Part model, mm, in its own coordinate system. A direction names the side the tool comes from. Round coordinates to 2 decimals unless told otherwise and drop trailing zeros. Loops run counter-clockwise (first coordinate to the right, second up) from the corner with the lowest first, then second, coordinate; pieces in that order, holes last. Notation, with made-up numbers: (67, -32.5) -> (94, -32.5) arc R7 ccw to (94, -21.5) -> close; hole circle Ø10 at (17.5, 22). An arc over 180 degrees is marked (long way). Use a Markdown table: item, result. Add a question column.
Item 1: Flat gauge pins, fed straight in: pin 1 (1.5 mm diameter, centred on x = -6.5, z = 1.5, fed in from +Y); pin 2 (2.5 mm diameter, centred on y = -28, z = 2, fed in from +X); pin 3 (2.5 mm diameter, centred on y = -7.5, z = 2, fed in from -X); pin 4 (12 mm diameter, centred on x = -17.5, y = -3, fed in from -Z). Where does each tip first touch, or does it go through?
Item 2: Cut at D-D, the plane x = -13.25. List the corners of the cut face in (y, z).
Item 3: Which spindle directions (+Z, -Z, +X, -X, +Y, -Y) get a long thin tool onto all of the face, cutting with end or side? Do faces 5 (the face through (-15, -10.262, 2)), 6 (the face through (-1.875, -28, 2)), 7 (the face through (-8.918, -28, 2)), 8 (the face through (-15.14, -15.42, 2.46)). Say none if no direction does.
Item 4: Two-plate mould, pull along X, no slides. Class faces 1 (the face through (-0.54, -2.44, 2.46)), 2 (the face through (-5.09, -36.07, 2.46)), 3 (the face through (-3, -14, 5)), 4 (the face through (1.61, -33.874, 2.465)): pulls with the +X half, pulls with the -X half, needs draft (parallel to the pull), parting line crosses it, or undercut.
Item 5: Cut at C-C, the plane x = -20.5. List the corners of the cut face in (y, z), plus the area to 3 significant figures.
Item 6: Cut at A-A, the plane x = 0. List the corners of the cut face in (y, z).
Item 7: Cut at B-B, the plane z = 1.2. List the corners of the cut face in (x, y), plus the area to 3 significant figures.
Item 8: Probe line 1 (Y direction, x = 0, z = 1.25); line 2 (X direction, y = -10, z = 0.85); line 3 (X direction, y = -26, z = 2.05). List the from-to ranges inside material, lowest first. Write a range as [from, to].
```python
from build123d import *

# Parameters (mm, degrees)
SKETCH_1_R      = 5
SKETCH_1_R_2    = 2.5
EXTRUDE_1_DEPTH = 5


with BuildPart() as part:
    # 스케치1 → 보스-돌출1 (new body)
    # profile 1 of 3: a face of its own
    with BuildSketch(Plane.XY):
        with BuildLine():
            ThreePointArc((-5, 0), (0, 5), (5, 0))
            Line((5, 0), (5, 15))
            Line((5, 15), (3.042493031, 15))
            Line((3.042493031, 15), (-5, 7.220187609))
            Line((-5, 7.220187609), (-5, 0))
        make_face()
    # profile 2 of 3: a face of its own
    with BuildSketch(Plane.XY):
        Circle(SKETCH_1_R)
        Circle(SKETCH_1_R_2, mode=Mode.SUBTRACT)
    # profile 3 of 3: a face of its own
    with BuildSketch(Plane.XY):
        with BuildLine():
            Line((5, -18.348194171), (5, 0))
            ThreePointArc((5, 0), (0, -5), (-5, 0))
            Line((-5, 0), (-4.999740664, -10.261800472))
            Line((-4.999740664, -10.261800472), (-25, -10.261800472))
            Line((-25, -10.261800472), (-25, -13.231879179))
            Line((-25, -13.231879179), (-5.003340767, -17.667219117))
            Line((-5.003340767, -17.667219117), (-8.918287267, -24.027561259))
            Line((-8.918287267, -24.027561259), (-8.918287267, -32.241958326))
            Line((-8.918287267, -32.241958326), (-1.160245593, -40))
            Line((-1.160245593, -40), (5, -40))
            Line((5, -40), (5, -37.263121262))
            Line((5, -37.263121262), (-1.875384477, -30.387736785))
            Line((-1.875384477, -30.387736785), (-1.875384477, -25.223578647))
            Line((-1.875384477, -25.223578647), (5, -18.348194171))
        make_face()
    extrude(amount=EXTRUDE_1_DEPTH)


solid = part.part
```
A:
| question | item | result |
|---|---|---|
| 1 | pin 1 | stops at y = -10.26 |
| 1 | pin 2 | stops at x = -1.88 |
| 1 | pin 3 | stops at x = -5 |
| 1 | pin 4 | passes through |
| 2 | outline | (-15.84, 0) -> (-10.26, 0) -> (-10.26, 5) -> (-15.84, 5) -> close |
| 3 | face 5 | +Z, -Z, -X, +Y |
| 3 | face 6 | +Z, -Z, +X |
| 3 | face 7 | +Z, -Z, -X, -Y |
| 3 | face 8 | +Z, -Z, -X |
| 4 | face 1 | undercut |
| 4 | face 2 | pulls with the -X half |
| 4 | face 3 | needs draft |
| 4 | face 4 | pulls with the +X half |
| 5 | outline | (-14.23, 0) -> (-10.26, 0) -> (-10.26, 5) -> (-14.23, 5) -> close |
| 5 | area | 19.8 mm^2 |
| 6 | outline | (-40, 0) -> (-32.26, 0) -> (-32.26, 5) -> (-40, 5) -> close; (-23.35, 0) -> (-2.5, 0) -> (-2.5, 5) -> (-23.35, 5) -> close; (2.5, 0) -> (12.06, 0) -> (12.06, 5) -> (2.5, 5) -> close |
| 7 | outline | (-25, -13.23) -> (-5, -17.67) -> (-8.92, -24.03) -> (-8.92, -32.24) -> (-1.16, -40) -> (5, -40) -> (5, -37.26) -> (-1.88, -30.39) -> (-1.88, -25.22) -> (5, -18.35) -> (5, 15) -> (3.04, 15) -> (-5, 7.22) -> (-5, 0) -> (-5, -10.26) -> (-25, -10.26) -> close; hole circle Ø5 at (0, 0) |
| 7 | area | 565 mm^2 |
| 8 | line 1 | y = [-40, -32.26], [-23.35, -2.5], [2.5, 12.06] |
| 8 | line 2 | x = [-5, 5] |
| 8 | line 3 | x = [-8.92, -1.88] |
